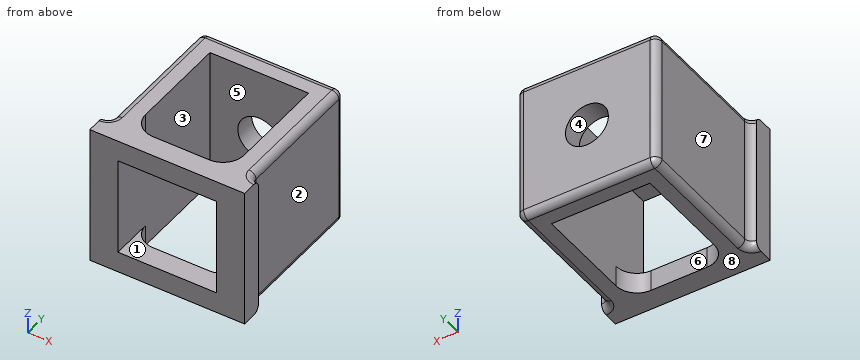
```python
from build123d import *

# Parameters (mm, degrees)
SKETCH_1_W      = 14
SKETCH_1_H      = 20
SKETCH_1_R      = 3.05
EXTRUDE_1_DEPTH = 3
EXTRUDE_2_DEPTH = 20
SKETCH_4_W      = 22
SKETCH_4_H      = 20
SKETCH_4_W_2    = 14
SKETCH_4_H_2    = 14
EXTRUDE_4_DEPTH = 3
FILLET_2_R      = 1
FILLET_3_R      = 3


with BuildPart() as part:
    # 草图1 → 凸台-拉伸1 (new body)
    with BuildSketch(Plane(origin=(0, 0, 0), x_dir=(1, 0, 0), z_dir=(0, 1, 0))):
        Rectangle(SKETCH_1_W, SKETCH_1_H)
        with Locations(Location((0, 0, 0), (0, 0, 270))):
            Circle(SKETCH_1_R, mode=Mode.SUBTRACT)
    extrude(amount=EXTRUDE_1_DEPTH)

    # 草图2 → 凸台-拉伸2 (add)
    with BuildSketch(Plane.XY.offset(10)):
        Polygon((-7, 3), (-7, 0), (-7, -20), (-11, -20), (-11, -17), (-10, -17), (-10, 0), (-10, 3), align=None)
        Polygon((10, 3), (10, 0), (10, -17), (11, -17), (11, -20), (7, -20), (7, 0), (7, 3), align=None)
    extrude(amount=-EXTRUDE_2_DEPTH)

    # 草图4 → 凸台-拉伸4 (add)
    with BuildSketch(Plane.XZ.offset(20)):
        Rectangle(SKETCH_4_W, SKETCH_4_H)
        Rectangle(SKETCH_4_W_2, SKETCH_4_H_2, mode=Mode.SUBTRACT)
    extrude(amount=-EXTRUDE_4_DEPTH)

    # 圆角2
    fillet_2_edges = [part.edges().sort_by_distance(p)[0] for p in [
        (-10, -17, 0),
        (10, -17, 0),
    ]]
    fillet(fillet_2_edges, radius=FILLET_2_R - 0.0001)  # a hair under: the kernel refuses the full size
    fillet_2_2_edges = [part.edges().sort_by_distance(p)[0] for p in [
        (-10, 3, 0),
        (0, 3, -10),
        (10, 3, 0),
        (0, 3, 10),
        (-10, -6.50005, -10),
        (-10, -6.50005, 10),
        (10, -6.50005, -10),
        (10, -6.50005, 10),
        (10.292863929, -16.707136071, 10),
        (10.292863929, -16.707136071, -10),
        (-10.292863929, -16.707136071, 10),
        (-10.292863929, -16.707136071, -10),
    ]]
    fillet(fillet_2_2_edges, radius=FILLET_2_R)

    # 圆角3
    fillet_3_edges = [part.edges().sort_by_distance(p)[0] for p in [
        (7, -17, -8.5),
        (7, -17, 8.5),
        (-7, -17, -8.5),
        (-7, -17, 8.5),
    ]]
    fillet(fillet_3_edges, radius=FILLET_3_R)


solid = part.part
```
Here's how the part is built. I have some questions about the finished solid (model axes, mm). Face numbers are marked on the shaded views. A direction names the side the tool comes from. Coordinates: 2 decimals unless noted, no trailing zeros. Write each loop counter-clockwise with the first axis right and the second up, starting at its lowest first coordinate (ties: lowest second). Pieces come first, ordered by that corner, then holes. Notation, with made-up numbers: (48, 47.25) -> (63, 47.25) arc R25 ccw to (63, 71.25) -> close; hole circle Ø4 at (6.25, 34). An arc over 180 degrees is marked (long way). Use a Markdown table: item, result. Add a question column.
(1) If we section it at A-A, the plane y = -13: Write out the boundary of the cut face in (x, z).
(2) For the marked faces 1, 2, 3, 4 and 5, which set-ups out of +Z, -Z, +X, -X, +Y, -Y let a thin tool reach every point of the face, with its end or its side?
(3) If we section it at D-D, the plane y = 1.25: Write out the boundary of the cut face in (x, z), and give its area (3 significant figures).
(4) Please list where these lines run through material, in increasing order: line 1 (X direction, y = 0.7, z = 0); line 2 (X direction, y = -4.75, z = 6.5); line 3 (Y direction, x = -6.25, z = -2).
(5) I'm going to push flat-ended pins straight in: P1, Ø8, axis at y = -11, z = 6, coming from the -X side; P2, Ø1, axis at y = -8.5, z = 0.5, coming from the +X side. Where does each tip first touch, or does it pass through?
(6) We'd pull the mould along X, two halves only. Please class the marked faces 6, 7 and 8: +X half, -X half, draft (parallel to the pull), parting line (faces both ways), or undercut.
(7) If we section it at B-B, the plane x = 0: Write out the boundary of the cut face in (y, z), and give its area (3 significant figures).
Outcome:
| question | item | result |
|---|---|---|
| 1 | outline | (-10, -9) arc R1 ccw to (-9, -10) -> (-7, -10) -> (-7, 10) -> (-9, 10) arc R1 ccw to (-10, 9) -> close; (7, -10) -> (9, -10) arc R1 ccw to (10, -9) -> (10, 9) arc R1 ccw to (9, 10) -> (7, 10) -> close |
| 2 | face 1 | -Y |
| 2 | face 2 | +Z, -Z, +X, +Y |
| 2 | face 3 | none |
| 2 | face 4 | +Y, -Y |
| 2 | face 5 | +Z, -Z |
| 3 | outline | (-10, -9) arc R1 ccw to (-9, -10) -> (9, -10) arc R1 ccw to (10, -9) -> (10, 9) arc R1 ccw to (9, 10) -> (-9, 10) arc R1 ccw to (-10, 9) -> close; hole circle Ø6.1 at (0, 0) |
| 3 | area | 370 mm^2 |
| 4 | line 1 | x = -10 to -3.05, 3.05 to 10 |
| 4 | line 2 | x = -10 to -7, 7 to 10 |
| 4 | line 3 | y = 0 to 3 |
| 5 | P1 | stops at x = -10 |
| 5 | P2 | stops at x = 10 |
| 6 | face 6 | undercut |
| 6 | face 7 | -X half |
| 6 | face 8 | draft |
| 7 | outline | (-20, -10) -> (-17, -10) -> (-17, -7) -> (-20, -7) -> close; (-20, 7) -> (-17, 7) -> (-17, 10) -> (-20, 10) -> close; (0, -10) -> (2, -10) arc R1 ccw to (3, -9) -> (3, -3.05) -> (0, -3.05) -> close; (0, 3.05) -> (3, 3.05) -> (3, 9) arc R1 ccw to (2, 10) -> (0, 10) -> close |
| 7 | area | 59.3 mm^2 |
